Autodesk Inventor part; units mm, degrees
ref_plane "Work Plane1" through (29, 0, 0) normal (0, -1, 0) x (1, 0, 0)
ref_plane "YZ Plane" through (0, 0, 0) normal (1, 0, 0) x (0, 1, 0)
ref_plane "XZ Plane" through (0, 0, 0) normal (0, 1, 0) x (-1, 0, 0)
sketch "Sketch1" plane through (0, 0, 0) normal (0, 0, 1) x (1, 0, 0)
  line L0 (-1.3333, 0) -> (100, 0)
  line L1 (100, 0) -> (100, 3)
  line L2 (100, 3) -> (76, 3)
  line L3 (76, 3) -> (75.3865, 3)
  line L4 (75.3865, 3) -> (0, 3)
  line L5 (0, 3) -> (0, 5)
  line L6 (0, 5) -> (-6, 5)
  line L7 (-6, 5) -> (-6, 2.8868)
  line L8 (-6, 2.8868) -> (-3, 2.8868)
  line L9 (-3, 2.8868) -> (-1.3333, 0)
  line L10 (-27.2, 0) -> (121.2, 0)
  line L11 (0, -1) -> (0, 6)
  line L12 (76, 3) -> (0, 3) construction
  dimension "d1" = 24
  dimension "d2" = 0.6136
  dimension "d3" = 6
  dimension "d4" = 3
  dimension "d5" = 60
  dimension "d6" = 6
  dimension "d7" = 6
  dimension "d8" = 5.7735
  dimension "d9" = 10
  dimension "d26" = 100
revolve "Body" add sketch "Sketch1" angle 360 about axis through (-1.3333, 0, 0) along (1, 0, 0)
sketch "Sketch2" plane through (-6, 0, 0) normal (-1, 0, 0) x (0, 0, 1)
  circle A0 centre (0, 0) radius 2.8868
  line L0 (0, -7) -> (0, 7)
  line L1 (-7, 0) -> (7, 0)
  line L2 (2.8868, 0) -> (1.4434, -2.5)
  line L3 (1.4434, -2.5) -> (-1.4434, -2.5)
  line L4 (-1.4434, -2.5) -> (-2.8868, 0)
  line L5 (-2.8868, 0) -> (-1.4434, 2.5)
  line L6 (-1.4434, 2.5) -> (1.4434, 2.5)
  line L7 (1.4434, 2.5) -> (2.8868, 0)
extrude "Slot" add sketch "Sketch2" against normal up to next contours L7 A0 | A0 L2 | L6 L0 A0 | A0 L0 L3 | L0 L6 A0 | A0 L3 L0 | L4 A0 | A0 L5
fillet "Fillet1" radius 0.4 1 edges at (-6, -5, 0)
thread "Thread"
chamfer "Chamfer1" distance 0.6135 distance2 0.6135 1 edges at (100, -3, 0) measured on face at (100, -0.7776, 0.9024)
ref_plane "Work Plane1" through (29, 0, 0) normal (0, -1, 0) x (1, 0, 0)
fillet "Fillet2" radius 0.1 1 edges at (0, -3, 0)
equation "\"d1\" = GEL"
equation "\"d3\" = KOH"
equation "\"d4\" = INTI"
equation "\"d6\" = GD"
equation "\"d7\" = BDM"
equation "\"d8\" = 1.1547 * SW"
equation "\"d9\" = KOD"
equation "\"d26\" = NLG"
equation "\"d30\" = R"
equation "\"d17\" = RR"
equation "\"d13\" = GEL"
equation "\"d15\" = -0.5 * SPD + 0.5 * GD"
equation "\"d16\" = GUL"
equation "\"GD\" = NND"
equation "\"NLG\" = 100"
equation "\"GEL\" = 24"
equation "\"KOD\" = 10"
equation "\"KOH\" = NND"
equation "\"INTI\" = 3"
equation "\"GAL\" = 0.61345 * PTC"
equation "\"GUL\" = 0.61345 * PTC"
equation "\"BDM\" = NND"
equation "\"SW\" = 5"
equation "\"RR\" = 0.4"
equation "\"SPD\" = NND - 1.2269 * PTC"
equation "\"R\" = 0.1"
equation "\"PHH\" = 0.1 * NND"
equation "\"GD1\" = THREADDIA - 1.2269 * PTC"
equation "\"THREADDIA\" = 6"
equation "\"FAWI\" = 45deg"
equation "\"PTC\" = 1"
equation "\"NND\" = 6"
equation "\"FAWI1\" = 30deg"
equation "\"TOA\" = 30deg"
equation "\"E0\" = 1.155 * SW"
properties part number "Unbrako - M6 x 100" material "Steel, Mild"
Geometry check sheet. Reference: the model listing, model coordinates, mm. A direction names the side the tool comes from. Coordinates: 2 decimals unless noted, no trailing zeros. Write each loop counter-clockwise with the first axis right and the second up, starting at its lowest first coordinate (ties: lowest second). Pieces come first, ordered by that corner, then holes. Notation, with made-up numbers: M -35.75,64.25 L -7.75,64.25 A20 cw -7.75,72.25 Z; hole C 18,-10.5 d5. An arc over 180 degrees is marked long. Use one line per item in the form item = value. Start each with the question number.
1) Section check A-A on x = 64. Enter the section's corners in (y, z).
2) Set-up check for faces 4 (the flat face through (-6, -2, 2)), 5 (the flat face through (0, 3.3, 0.1)), 6 (the flat face through (-4.411, -1.233, 2.175)): record each of +Z, -Z, +X, -X, +Y, -Y from which the full face is reachable in a straight line by a thin tool's end or side.
3) Release check for a two-part mould opening along Z. For faces 1 (the flat face through (-4.411, -1.268, -2.155)), 2 (the flat face through (100, 0, 0)), 3 (the cylindrical face through (49, -3, 0)) record: pulls with the +Z half, pulls with the -Z half, needs draft (parallel to the pull), parting line crosses it, or undercut.
4) Thickness scan on probe 1 along X at (y, z) = (-3, 3.25); probe 2 along Y at (x, z) = (70, -0.75); probe 3 along Y at (x, z) = (23, -0.25). Record the ranges inside material, lowest first. Write a range as from..to.
5) Go/stop test with flat-tipped pins: pin 1 Ø1.5 at (x, z) = (22, 3) entering from +Y; pin 2 Ø1 at (x, z) = (43.5, 2.5) entering from +Y; pin 3 Ø3 at (x, z) = (-4.5, 0.5) entering from -Y; pin 4 Ø6 at (x, z) = (63, 3) entering from +Y. Record where each tip stops, or that it passes through.
Responses:
q1.outline = C 0,0 d6
q2.face_4 = +Z, -Z, -X, +Y, -Y
q2.face_5 = +X
q2.face_6 = -X
q3.face_1 = undercut
q3.face_2 = needs draft
q3.face_3 = parting line crosses it
q4.probe_1 = -6..0
q4.probe_2 = -2.9..2.9
q4.probe_3 = -2.99..2.99
q5.pin_1 = 1.98
q5.pin_2 = 2.24
q5.pin_3 = -5
q5.pin_4 = 3
